```python
from build123d import *

# Parameters (mm, degrees)
SKETCH_W  = 200
SKETCH_H  = 120
SKETCH_R  = 2.5
PAD_DEPTH = 1.8


with BuildPart() as part:
    # Sketch → Pad (new body)
    with BuildSketch(Plane.XY):
        with Locations((90, 55.5)):
            Rectangle(SKETCH_W, SKETCH_H)
        Circle(SKETCH_R, mode=Mode.SUBTRACT)
        with Locations((0, 20)):
            Circle(SKETCH_R, mode=Mode.SUBTRACT)
        with Locations((0, 40)):
            Circle(SKETCH_R, mode=Mode.SUBTRACT)
        with Locations((0, 60)):
            Circle(SKETCH_R, mode=Mode.SUBTRACT)
        with Locations((20, 10)):
            Circle(SKETCH_R, mode=Mode.SUBTRACT)
        with Locations((20, 30)):
            Circle(SKETCH_R, mode=Mode.SUBTRACT)
        with Locations((20, 50)):
            Circle(SKETCH_R, mode=Mode.SUBTRACT)
        with Locations((20, 70)):
            Circle(SKETCH_R, mode=Mode.SUBTRACT)
        with Locations((40, 0)):
            Circle(SKETCH_R, mode=Mode.SUBTRACT)
        with Locations((40, 20)):
            Circle(SKETCH_R, mode=Mode.SUBTRACT)
        with Locations((40, 40)):
            Circle(SKETCH_R, mode=Mode.SUBTRACT)
        with Locations((40, 60)):
            Circle(SKETCH_R, mode=Mode.SUBTRACT)
        with Locations((60, 10)):
            Circle(SKETCH_R, mode=Mode.SUBTRACT)
        with Locations((60, 30)):
            Circle(SKETCH_R, mode=Mode.SUBTRACT)
        with Locations((60, 50)):
            Circle(SKETCH_R, mode=Mode.SUBTRACT)
        with Locations((60, 70)):
            Circle(SKETCH_R, mode=Mode.SUBTRACT)
        with Locations((80, 0)):
            Circle(SKETCH_R, mode=Mode.SUBTRACT)
        with Locations((80, 20)):
            Circle(SKETCH_R, mode=Mode.SUBTRACT)
        with Locations((80, 40)):
            Circle(SKETCH_R, mode=Mode.SUBTRACT)
        with Locations((80, 60)):
            Circle(SKETCH_R, mode=Mode.SUBTRACT)
        with Locations((100, 10)):
            Circle(SKETCH_R, mode=Mode.SUBTRACT)
        with Locations((100, 30)):
            Circle(SKETCH_R, mode=Mode.SUBTRACT)
        with Locations((100, 50)):
            Circle(SKETCH_R, mode=Mode.SUBTRACT)
        with Locations((100, 70)):
            Circle(SKETCH_R, mode=Mode.SUBTRACT)
        with Locations((120, 0)):
            Circle(SKETCH_R, mode=Mode.SUBTRACT)
        with Locations((120, 20)):
            Circle(SKETCH_R, mode=Mode.SUBTRACT)
        with Locations((120, 40)):
            Circle(SKETCH_R, mode=Mode.SUBTRACT)
        with Locations((120, 60)):
            Circle(SKETCH_R, mode=Mode.SUBTRACT)
        with Locations((140, 10)):
            Circle(SKETCH_R, mode=Mode.SUBTRACT)
        with Locations((140, 30)):
            Circle(SKETCH_R, mode=Mode.SUBTRACT)
        with Locations((140, 50)):
            Circle(SKETCH_R, mode=Mode.SUBTRACT)
        with Locations((140, 70)):
            Circle(SKETCH_R, mode=Mode.SUBTRACT)
        with Locations((160, 0)):
            Circle(SKETCH_R, mode=Mode.SUBTRACT)
        with Locations((160, 20)):
            Circle(SKETCH_R, mode=Mode.SUBTRACT)
        with Locations((160, 40)):
            Circle(SKETCH_R, mode=Mode.SUBTRACT)
        with Locations((160, 60)):
            Circle(SKETCH_R, mode=Mode.SUBTRACT)
        with Locations((180, 10)):
            Circle(SKETCH_R, mode=Mode.SUBTRACT)
        with Locations((180, 30)):
            Circle(SKETCH_R, mode=Mode.SUBTRACT)
        with Locations((180, 50)):
            Circle(SKETCH_R, mode=Mode.SUBTRACT)
        with Locations((180, 70)):
            Circle(SKETCH_R, mode=Mode.SUBTRACT)
        with Locations((0, 80)):
            Circle(SKETCH_R, mode=Mode.SUBTRACT)
        with Locations((20, 90)):
            Circle(SKETCH_R, mode=Mode.SUBTRACT)
        with Locations((40, 80)):
            Circle(SKETCH_R, mode=Mode.SUBTRACT)
        with Locations((60, 90)):
            Circle(SKETCH_R, mode=Mode.SUBTRACT)
        with Locations((80, 80)):
            Circle(SKETCH_R, mode=Mode.SUBTRACT)
        with Locations((100, 90)):
            Circle(SKETCH_R, mode=Mode.SUBTRACT)
        with Locations((120, 80)):
            Circle(SKETCH_R, mode=Mode.SUBTRACT)
        with Locations((140, 90)):
            Circle(SKETCH_R, mode=Mode.SUBTRACT)
        with Locations((160, 80)):
            Circle(SKETCH_R, mode=Mode.SUBTRACT)
        with Locations((180, 90)):
            Circle(SKETCH_R, mode=Mode.SUBTRACT)
        with Locations((0, 100)):
            Circle(SKETCH_R, mode=Mode.SUBTRACT)
        with Locations((40, 100)):
            Circle(SKETCH_R, mode=Mode.SUBTRACT)
        with Locations((80, 100)):
            Circle(SKETCH_R, mode=Mode.SUBTRACT)
        with Locations((120, 100)):
            Circle(SKETCH_R, mode=Mode.SUBTRACT)
        with Locations((160, 100)):
            Circle(SKETCH_R, mode=Mode.SUBTRACT)
        with Locations((20, 110)):
            Circle(SKETCH_R, mode=Mode.SUBTRACT)
        with Locations((60, 110)):
            Circle(SKETCH_R, mode=Mode.SUBTRACT)
        with Locations((100, 110)):
            Circle(SKETCH_R, mode=Mode.SUBTRACT)
        with Locations((140, 110)):
            Circle(SKETCH_R, mode=Mode.SUBTRACT)
        with Locations((180, 110)):
            Circle(SKETCH_R, mode=Mode.SUBTRACT)
    extrude(amount=PAD_DEPTH)


solid = part.part
```
For this review, take the finished solid that the model builds, in its own axes (mm). Round coordinates to 2 decimals unless told otherwise and drop trailing zeros. Loops run counter-clockwise (first coordinate to the right, second up) from the corner with the lowest first, then second, coordinate; pieces in that order, holes last.
(1) Clearance check with a flat-ended pin moving along its axis: P1, Ø3, axis at x = 0, y = 80, coming from the -Z side. State where the tip first meets the part, or that it passes through.
Returned:
P1: passes through
(2) We need section A-A (y = 80). Give the boundary of the cut face in (x, z).
Returned:
outline: (-10, 0) - (-2.5, 0) - (-2.5, 1.8) - (-10, 1.8) - close; (2.5, 0) - (37.5, 0) - (37.5, 1.8) - (2.5, 1.8) - close; (42.5, 0) - (77.5, 0) - (77.5, 1.8) - (42.5, 1.8) - close; (82.5, 0) - (117.5, 0) - (117.5, 1.8) - (82.5, 1.8) - close; (122.5, 0) - (157.5, 0) - (157.5, 1.8) - (122.5, 1.8) - close; (162.5, 0) - (190, 0) - (190, 1.8) - (162.5, 1.8) - close
(3) We need section B-B (x = 60). Give the boundary of the cut face in (y, z), plus the area to 3 significant figures.
Returned:
outline: (-4.5, 0) - (7.5, 0) - (7.5, 1.8) - (-4.5, 1.8) - close; (12.5, 0) - (27.5, 0) - (27.5, 1.8) - (12.5, 1.8) - close; (32.5, 0) - (47.5, 0) - (47.5, 1.8) - (32.5, 1.8) - close; (52.5, 0) - (67.5, 0) - (67.5, 1.8) - (52.5, 1.8) - close; (72.5, 0) - (87.5, 0) - (87.5, 1.8) - (72.5, 1.8) - close; (92.5, 0) - (107.5, 0) - (107.5, 1.8) - (92.5, 1.8) - close; (112.5, 0) - (115.5, 0) - (115.5, 1.8) - (112.5, 1.8) - close
area: 162 mm2
(4) We need section C-C (z = 0.4). State how many separate pieces and enclosed holes the cut face has, plus the area to 3 significant figures.
Returned:
separate pieces: 1
enclosed holes: 60
area: 22,800 mm2
(5) Wall thickness on line 1 along X through (y, z) = (29.5, 1.3); line 2 along X through (y, z) = (91.5, 1.3): over which ranges is each line inside the solid? List them lowest first.
Returned:
line 1: x = -10 to 17.55, 22.45 to 57.55, 62.45 to 97.55, 102.45 to 137.55, 142.45 to 177.55, 182.45 to 190
line 2: x = -10 to 18, 22 to 58, 62 to 98, 102 to 138, 142 to 178, 182 to 190
